Geometry check sheet. Reference: the model listing, model coordinates, mm. Give positions to 0.01 mm unless a question says otherwise; leave off trailing zeros. Loops run counter-clockwise (first coordinate to the right, second up) from the corner with the lowest first, then second, coordinate; pieces in that order, holes last.
1. Cross-section at D-D, the plane y = 70.5. Record the cut outline in (x, z), plus the area to 3 significant figures.
2. Cross-section at A-A, the plane x = 38. Record the cut outline in (y, z) (1 decimal).
3. Go/stop test with flat-tipped pins: pin 1 Ø3.5 at (x, y) = (45.5, 69.5) entering from -Z; pin 2 Ø4 at (x, z) = (30.5, 38.5) entering from -Y. Record where each tip stops, or that it passes through.
4. Material ranges on L1, parallel to X at y = 23.5, z = 20; L2, parallel to Y at x = 39, z = 7.5; L3, parallel to X at y = 26.5, z = 29, recorded low to high.
5. Cross-section at C-C, the plane z = 79.5. Record the cut outline in (x, y) (3 decimals), plus the area to 3 significant figures.
6. Cross-section at B-B, the plane z = 15. Record the cut outline in (x, y).
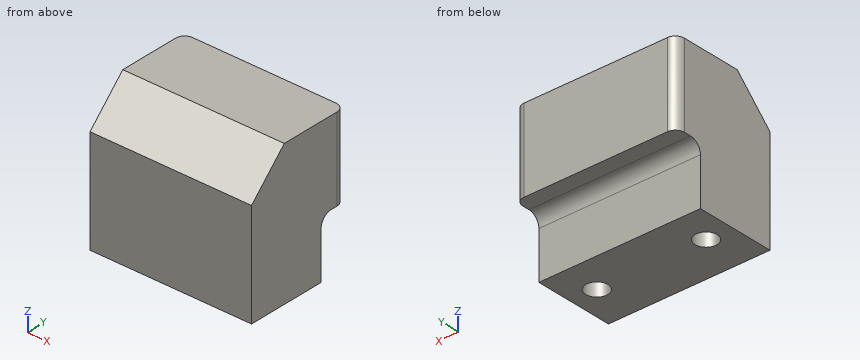
from build123d import *

# Parameters (mm, degrees)
F1_DEPTH = 112.6998
F3_D     = 15.4432
F3_DEPTH = 38.1
F3_TIP   = 4.6396053559
F4_R     = 6.35
F5_R     = 7.9375


with BuildPart() as f1:
    # F0 (on Right) → F1 (new body)
    with BuildSketch(Plane.YZ):
        Polygon((74.5998005843, 99.187), (26.162, 99.187), (0, 73.025), (0, 0), (55.5625, 0), (55.5497996769, 41.148), (74.5998005843, 41.148), align=None)
    extrude(amount=F1_DEPTH)

    # F3
    with Locations(Plane(origin=(0, 0, 0), x_dir=(1, 0, 0), z_dir=(0, 0, -1))):
        with Locations((94.4626, -30.1625), (18.2626, -30.1625)):
            Hole(F3_D / 2, depth=F3_DEPTH)
            with Locations((0, 0, -(F3_DEPTH + F3_TIP / 2))):  # 118° drill point
                Cone(0, F3_D / 2, F3_TIP, mode=Mode.SUBTRACT)

    # F4
    f4_edges = [f1.edges().sort_by_distance(p)[0] for p in [
        (112.6998, 74.599801, 70.1675),
        (0, 74.599801, 70.1675),
    ]]
    fillet(f4_edges, radius=F4_R)

    # F5
    f5_edges = [f1.edges().sort_by_distance(p)[0] for p in [
        (56.3499, 55.5498, 41.148),
    ]]
    fillet(f5_edges, radius=F5_R)


solid = f1.part
Result:
1. outline: (0.41, 41.15) - (112.29, 41.15) - (112.29, 99.19) - (0.41, 99.19) - close
1. area: 6,490 mm2
2. outline: (0, 0) - (55.6, 0) - (55.6, 33.2) arc R7.9 cw to (63.5, 41.1) - (74.6, 41.1) - (74.6, 99.2) - (26.2, 99.2) - (0, 73) - close
3. pin 1: stops at z = 41.15
3. pin 2: stops at y = 0
4. L1: x = 0 to 14.36, 22.17 to 90.56, 98.37 to 112.7
4. L2: y = 0 to 55.56
4. L3: x = 0 to 11.46, 25.06 to 87.66, 101.26 to 112.7
5. outline: (0, 6.475) - (112.7, 6.475) - (112.7, 68.25) arc R6.35 ccw to (106.35, 74.6) - (6.35, 74.6) arc R6.35 ccw to (0, 68.25) - close
5. area: 7,660 mm2
6. outline: (0, 0) - (112.7, 0) - (112.7, 55.56) - (0, 55.56) - close; hole circle Ø15.44 at (18.26, 30.16); hole circle Ø15.44 at (94.46, 30.16)
